CAD build for the part. Positions are in the model's coordinates, mm. A direction names the side the tool comes from. Round coordinates to 2 decimals unless told otherwise and drop trailing zeros. Order: outer loops, then holes, each group sorted by start corner. A loop starts at its lowest first (then second) coordinate and runs counter-clockwise, first axis right, second up. Notation, with made-up numbers: M 5,86.5 L 21,86.5 A27 ccw 21,110.5 Z; hole C 87.5,16 d2. An arc over 180 degrees is marked long. Answer as CSV lines item,"result". Start each with the question number.
```python
from build123d import *

# Parameters (mm, degrees)
BOSS_EXTRUDE1_DEPTH = 101.6
CUT_EXTRUDE2_DEPTH  = 101.6
SKETCH5_R           = 1.651
CUT_EXTRUDE3_DEPTH  = 13.5992
FILLET1_R           = 2.54


with BuildPart() as part:
    # Sketch1 → Boss-Extrude1 (new body)
    with BuildSketch(Plane(origin=(0, 0, 0), x_dir=(0, 0, -1), z_dir=(1, 0, 0))):
        with BuildLine():
            Line((0, 16.7996), (0, 3.2004))
            Line((0, 3.2004), (9.525, 3.2004))
            Line((9.525, 3.2004), (9.525, 0))
            Line((9.525, 0), (14.605, 0))
            ThreePointArc((14.605, 0), (15.279774052, 1.174548121), (15.868724182, 2.394392806))
            Line((15.868724182, 2.394392806), (23.603930172, 20))
            Line((23.603930172, 20), (9.525, 20))
            Line((9.525, 20), (9.525, 16.7996))
            Line((9.525, 16.7996), (0, 16.7996))
        make_face()
    extrude(amount=BOSS_EXTRUDE1_DEPTH)

    # Sketch4 → Cut-Extrude2 (cut)
    with BuildSketch(Plane.ZY):
        with BuildLine():
            Line((0, 13.526281186), (0, 6.473718814))
            ThreePointArc((0, 6.473718814), (-2.36728, 10), (0, 13.526281186))
        make_face()
    extrude(amount=-CUT_EXTRUDE2_DEPTH, mode=Mode.SUBTRACT)

    # Sketch5 → Cut-Extrude3 (cut)
    with BuildSketch(Plane(origin=(0, 16.7996, 0), x_dir=(1, 0, 0), z_dir=(0, 1, 0))):
        with Locations((19.05, 4.7625)):
            Circle(SKETCH5_R)
        with Locations((82.55, 4.7625)):
            Circle(SKETCH5_R)
    extrude(amount=-CUT_EXTRUDE3_DEPTH, mode=Mode.SUBTRACT)

    # Fillet1
    fillet1_edges = [part.edges().sort_by_distance(p)[0] for p in [
        (50.8, 20, -23.603930172),
        (50.8, 0, -14.605),
    ]]
    fillet(fillet1_edges, radius=FILLET1_R)


solid = part.part
```
Q1. Mould opens along Y. For faces 4 (the cylindrical face through (84.075, 10.095, -4.13)), 5 (the cylindrical face through (50.089, 9.937, -2.367)), 6 (the cylindrical face through (51.511, 0.383, -14.469)), 7 (the flat face through (50, 20, -15)) say: +Y half, -Y half, draft (parallel to the pull), parting line (faces both ways), or undercut.
Q2. Band-saw the part on A-A, the plane x = 19.05. Write the cut outline in (y, z) (1 decimal).
Q3. Probe line 1 along X through (y, z) = (10.75, -4.75); line 2 along Z through (x, y) = (82.55, 7); line 3 along Y through (x, z) = (12, -4). List the from-to ranges inside material, lowest first. Write a range as from..to.
Q4. Band-saw the part on D-D, the plane x = 82.5. Write the cut outline in (y, z) (3 decimals), then the cut area to 3 significant figures.
Q5. Drop flat-ended pins along their axis: P1, Ø1, axis at x = 89.5, z = -6.5, coming from the -Y side; P2, Ø1, axis at x = 42, y = 9, coming from the +Z side; P3, Ø10.5, axis at x = 38, z = -3, coming from the +Y side. Give the stop position or say it passes through.
Q6. Tool access for faces 1 (the cylindrical face through (51.51, 18.88, -21.82)), 2 (the flat face through (50, 3.2, -5)), 3 (the flat face through (50, 18, -9.525)): list every direction of +Z, -Z, +X, -X, +Y, -Y with a clear straight run to the whole face (end or side of a thin tool).
Q7. Band-saw the part on B-B, the plane y = 10.5. Write the cut outline in (x, z).
Q8. Band-saw the part on C-C, the plane x = 38.5. Write the cut outline in (y, z) (3 decimals), then the cut area to 3 significant figures.
Answer:
1,face 4,"draft"
1,face 5,"undercut"
1,face 6,"-Y half"
1,face 7,"+Y half"
2,outline,"M 0,-13.1 A2.5 ccw 1.4,-15.4 A18.9 ccw 2.4,-15.9 L 16.4,-22 A2.5 ccw 20,-19.7 L 20,-9.5 L 16.8,-9.5 L 16.8,-6.4 L 3.2,-6.4 L 3.2,-9.5 L 0,-9.5 Z; M 3.2,-3.1 L 16.8,-3.1 L 16.8,0 L 13.5,0 A3.8 cw 6.5,0 L 3.2,0 Z"
3,line 1,"x = 0..17.4, 20.7..80.9, 84.2..101.6"
3,line 2,"z = -17.89..-6.41, -3.11..-0.91"
3,line 3,"y = 3.2..16.8"
4,outline,"M 0,-13.127 A2.54 ccw 1.382,-15.388 A18.908 ccw 2.394,-15.869 L 16.438,-22.039 A2.54 ccw 20,-19.714 L 20,-9.525 L 16.8,-9.525 L 16.8,-6.413 L 3.2,-6.413 L 3.2,-9.525 L 0,-9.525 Z; M 3.2,-3.112 L 16.8,-3.112 L 16.8,0 L 13.526,0 A3.81 cw 6.474,0 L 3.2,0 Z"
4,area,"262 mm^2"
5,P1,"stops at y = 3.2"
5,P2,"stops at z = -2.06"
5,P3,"stops at y = 16.8"
6,face 1,"-Z, +X, -X"
6,face 2,"+Z, +X, -X, -Y"
6,face 3,"+Z, +X, -X, +Y"
7,outline,"M 0,-19.43 L 101.6,-19.43 L 101.6,-2.33 L 0,-2.33 Z; hole C 19.05,-4.76 d3.3; hole C 82.55,-4.76 d3.3"
8,outline,"M 0,-13.127 A2.54 ccw 1.382,-15.388 A18.908 ccw 2.394,-15.869 L 16.438,-22.039 A2.54 ccw 20,-19.714 L 20,-9.525 L 16.8,-9.525 L 16.8,0 L 13.526,0 A3.81 cw 6.474,0 L 3.2,0 L 3.2,-9.525 L 0,-9.525 Z"
8,area,"307 mm^2"
